Could you check a few things on this drawing? It's one solid part, dimensions in mm from its lowest x, y, z. Coordinates: 2 decimals unless noted, no trailing zeros. Order: outer loops, then holes, each group sorted by start corner. A loop starts at its lowest first (then second) coordinate and runs counter-clockwise, first axis right, second up. Notation, with made-up numbers: M 10.25,-15.75 L 32.25,-15.75 A20 ccw 32.25,8.25 Z; hole C -23,82.25 d8. An arc over 180 degrees is marked long. Answer as CSV lines item,"result". Start each with the question number.
1. If we section it at A-A (z = 45): List the corners of the cut face in (x, y) for me, plus the area to 3 significant figures.
2. If we section it at B-B (y = 9.5): List the corners of the cut face in (x, z) for me.
3. Will these pins go through, and if not, where does the flat tip stop? pin 1 (14.5 mm diameter, centred on x = 97, y = 67, fed in from +Z); pin 2 (3 mm diameter, centred on x = 48, z = 25.5, fed in from -Y); pin 3 (3 mm diameter, centred on x = 151, y = 42.5, fed in from -Z).
4. If we section it at C-C (x = 50): List the corners of the cut face in (y, z) for me, plus the area to 3 significant figures.
5. If we section it at D-D (y = 40): List the corners of the cut face in (x, z) for me, plus the area to 3 significant figures.
6. I need wall thicknesses on line 1 along Y through (x, z) = (50, 5.5); line 2 along Y through (x, z) = (100, 47.25); line 3 along Z through (x, y) = (150, 10.75). Which ranges of each line are inside material? Lowest first, please. Write a range as from..to.
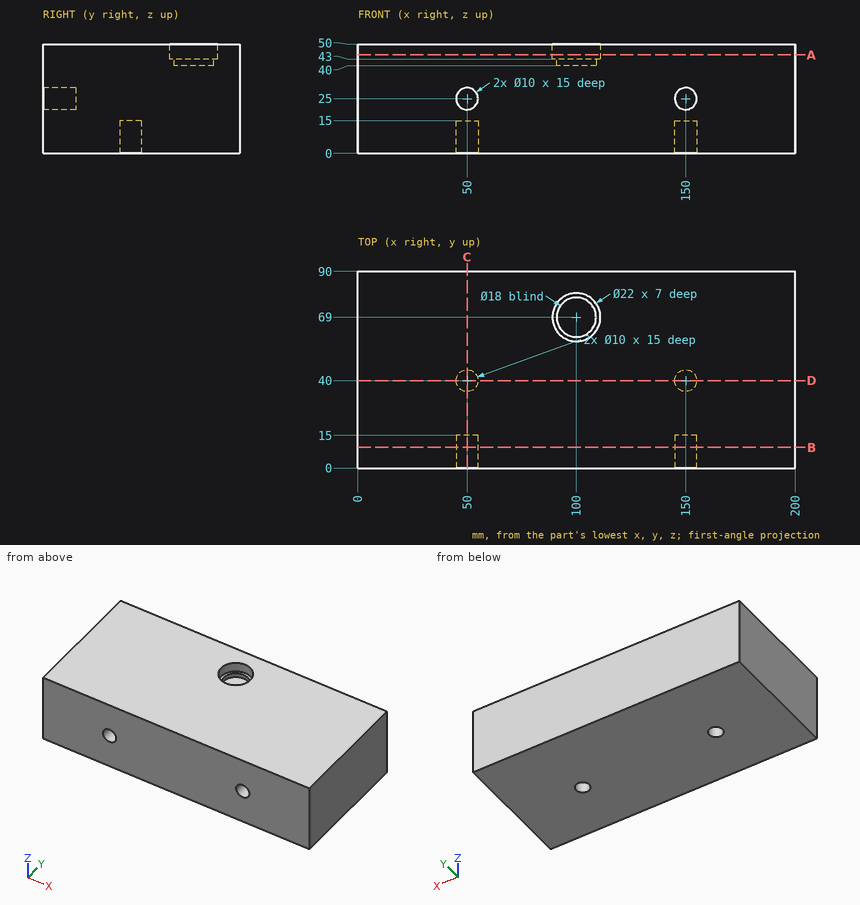
Solved:
1,outline,"M 0,0 L 200,0 L 200,90 L 0,90 Z; hole C 100,69 d22"
1,area,"17,600 mm²"
2,outline,"M 0,0 L 200,0 L 200,50 L 0,50 Z; hole C 50,25 d10; hole C 150,25 d10"
3,pin 1,"z = 43"
3,pin 2,"y = 15"
3,pin 3,"z = 15"
4,outline,"M 0,0 L 35,0 L 35,15 L 45,15 L 45,0 L 90,0 L 90,50 L 0,50 L 0,30 L 15,30 L 15,20 L 0,20 Z"
4,area,"4,200 mm²"
5,outline,"M 0,0 L 45,0 L 45,15 L 55,15 L 55,0 L 145,0 L 145,15 L 155,15 L 155,0 L 200,0 L 200,50 L 0,50 Z"
5,area,"9,700 mm²"
6,line 1,"0..35, 45..90"
6,line 2,"0..58, 80..90"
6,line 3,"0..20, 30..50"
